The drawing under review shows one solid part. Ordinate dimensions are in mm from its lowest x, y, z. Coordinates: 2 decimals unless noted, no trailing zeros. Loops run counter-clockwise (first coordinate to the right, second up) from the corner with the lowest first, then second, coordinate; pieces in that order, holes last. Notation, with made-up numbers: (17, 32.25) -> (42, 32.25) arc R25 ccw to (42, 50.25) -> close; hole circle Ø10 at (48, 79.5). An arc over 180 degrees is marked (long way). Use a Markdown table: item, result.
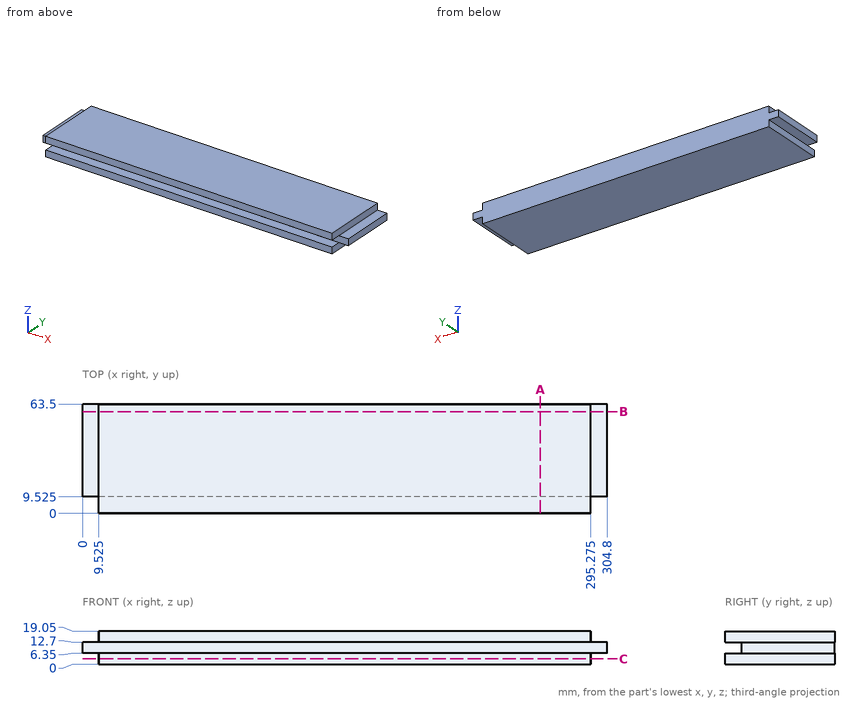
(1) Take a section at C-C on z = 3. Write out the cut boundary in (x, y) (3 decimals).
Found:
| item | result |
|---|---|
| outline | (9.525, 0) -> (295.275, 0) -> (295.275, 63.5) -> (9.525, 63.5) -> close |
(2) Take a section at B-B on y = 59. Write out the cut boundary in (x, z) (3 decimals).
Found:
| item | result |
|---|---|
| outline | (0, 6.35) -> (9.525, 6.35) -> (9.525, 0) -> (295.275, 0) -> (295.275, 6.35) -> (304.8, 6.35) -> (304.8, 12.7) -> (295.275, 12.7) -> (295.275, 19.05) -> (9.525, 19.05) -> (9.525, 12.7) -> (0, 12.7) -> close |
(3) For line 1 along Z through (x, y) = (154.5, 9); line 2 along X through (y, z) = (20, 14.25) (3 decimals); line 3 along Y through (x, z) = (85.5, 7.5) (3 decimals), list the stretches that pass through material, from the lowest coordinate up.
Found:
| item | result |
|---|---|
| line 1 | z = 0 to 6.35, 12.7 to 19.05 |
| line 2 | x = 9.525 to 295.275 |
| line 3 | y = 9.525 to 63.5 |
(4) For pin 1 Ø1.9 at (y, z) = (29.5, 3.5) entering from -X (3 decimals); pin 2 Ø5 at (x, y) = (299, 37) entering from -Z; pin 3 Ø10.5 at (x, y) = (301, 46) entering from +Z, all flat-tipped, find the tip position at first contact; note any pin that passes through.
Found:
| item | result |
|---|---|
| pin 1 | stops at x = 9.525 |
| pin 2 | stops at z = 6.35 |
| pin 3 | stops at z = 12.7 |
(5) Take a section at A-A on x = 266. Write out the cut boundary in (y, z) (3 decimals).
Found:
| item | result |
|---|---|
| outline | (0, 0) -> (63.5, 0) -> (63.5, 19.05) -> (0, 19.05) -> (0, 12.7) -> (9.525, 12.7) -> (9.525, 6.35) -> (0, 6.35) -> close |
